Geometry: final body of the model. Coordinates: model frame, mm. A direction names the side the tool comes from. Give positions to 0.01 mm unless a question says otherwise; leave off trailing zeros. Loops run counter-clockwise (first coordinate to the right, second up) from the corner with the lowest first, then second, coordinate; pieces in that order, holes last. Notation, with made-up numbers: (-11, 53) - (2, 53) arc R12 ccw to (2, 69) - close; hole circle Ø1 at (75.5, 48.5). An arc over 180 degrees is marked (long way). Use CSV: the item, a comma, the result in double quotes. Start each with the question number.
```python
from build123d import *

# Parameters (mm, degrees)
BOSS_EXTRU_1_DEPTH      = 6
BOSS_EXTRU_2_DEPTH      = 12
ESQUISSE14_W            = 21
ESQUISSE14_H            = 6
ENL_V_MAT_EXTRU_2_DEPTH = 21
D_GAGEMENT_M81_D        = 9
TROU_TARAUD_M82_D       = 6.8
ESQUISSE19_W            = 31.228123836
ESQUISSE19_H            = 16.033363116
ENL_V_MAT_EXTRU_3_DEPTH = 22
ESQUISSE20_W            = 8
ESQUISSE20_H            = 6
BOSS_EXTRU_3_DEPTH      = 25
BOSS_EXTRU_4_DEPTH      = 6
TROU_TARAUD_M83_D       = 6.8
ESQUISSE25_W            = 25
ESQUISSE25_H            = 6
ENL_V_MAT_EXTRU_4_DEPTH = 3
ENL_V_START             = -13
ENL_V_MAT_EXTRU_5_DEPTH = 14


with BuildPart() as part:
    # Esquisse1 → Boss.-Extru.1 (new body)
    with BuildSketch(Plane(origin=(0, 0, 0), x_dir=(1, 0, 0), z_dir=(0, 1, 0))):
        with BuildLine():
            Line((0, 0), (0, 30))
            ThreePointArc((0, 30), (10, 40), (20, 30))
            Line((20, 30), (20, 0))
            ThreePointArc((20, 0), (10, -10), (0, 0))
        make_face()
    extrude(amount=BOSS_EXTRU_1_DEPTH)

    # Esquisse12 → Boss.-Extru.2 (add)
    with BuildSketch(Plane.XZ):
        with BuildLine():
            Line((0, -30), (20, -30))
            Line((20, -30), (20, 0))
            ThreePointArc((20, 0), (10, 10), (0, 0))
            Line((0, 0), (0, -30))
        make_face()
    extrude(amount=BOSS_EXTRU_2_DEPTH)

    # Esquisse14 → Enlèv. mat.-Extru.2 (cut, through all)
    with BuildSketch(Plane(origin=(20, 0, 0), x_dir=(0, 0, -1), z_dir=(1, 0, 0))):
        with Locations((0.5, 3)):
            Rectangle(ESQUISSE14_W, ESQUISSE14_H)
        Polygon((30, 0), (19, 0), (19, -6), (-10, -6), (-10, -12), (30, -12), align=None)
    extrude(amount=-ENL_V_MAT_EXTRU_2_DEPTH, mode=Mode.SUBTRACT)

    # Dégagement M81 (through all)
    with Locations(Plane(origin=(0, 6, 0), x_dir=(1, 0, 0), z_dir=(0, 1, 0))):
        with Locations((10, 30)):
            Hole(D_GAGEMENT_M81_D / 2)

    # Trou taraudé M82 (through all)
    with Locations(Plane(origin=(0, 0, 0), x_dir=(1, 0, 0), z_dir=(0, 1, 0))):
        with Locations((10, 0)):
            Hole(TROU_TARAUD_M82_D / 2)

    # Esquisse19 → Enlèv. mat.-Extru.3 (cut, through all)
    with BuildSketch(Plane.XY.offset(-11)):
        with Locations((8.695037224, -0.70266631)):
            Rectangle(ESQUISSE19_W, ESQUISSE19_H)
    extrude(amount=ENL_V_MAT_EXTRU_3_DEPTH, mode=Mode.SUBTRACT)

    # Esquisse20 → Boss.-Extru.3 (add)
    with BuildSketch(Plane.ZY):
        with Locations((-15, -3)):
            Rectangle(ESQUISSE20_W, ESQUISSE20_H)
    extrude(amount=BOSS_EXTRU_3_DEPTH)

    # Esquisse21 → Boss.-Extru.4 (add)
    with BuildSketch(Plane.XZ.offset(6)):
        with BuildLine():
            Line((-25, -19), (-25, -30))
            ThreePointArc((-25, -30), (-15, -40), (-5, -30))
            Line((-5, -30), (-5, -19))
            Line((-5, -19), (-25, -19))
        make_face()
    extrude(amount=-BOSS_EXTRU_4_DEPTH)

    # Trou taraudé M83 (through all)
    with Locations(Plane(origin=(0, 0, 0), x_dir=(1, 0, 0), z_dir=(0, 1, 0))):
        with Locations((-15, 30)):
            Hole(TROU_TARAUD_M83_D / 2)

    # Esquisse25 → Enlèv. mat.-Extru.4 (cut)
    with BuildSketch(Plane(origin=(0, 0, -19), x_dir=(-1, 0, 0), z_dir=(0, 0, -1))):
        with Locations((-7.5, -3)):
            Rectangle(ESQUISSE25_W, ESQUISSE25_H)
    extrude(amount=-ENL_V_MAT_EXTRU_4_DEPTH, mode=Mode.SUBTRACT)

    # Esquisse27 → Enlèv. mat.-Extru.5 (cut)
    with BuildSketch(Plane.XZ.offset(6).offset(ENL_V_START)):
        Polygon((-25, -11), (-10, -11), (-25, -23.586494468), align=None)
    enl_v_mat_extru_5 = extrude(amount=ENL_V_MAT_EXTRU_5_DEPTH, mode=Mode.SUBTRACT)

    # Symétrie1: Enlèv. mat.-Extru.5 across plane
    add(enl_v_mat_extru_5.mirror(Plane(origin=(-2.5, 0, 0), x_dir=(0, 0, 1), z_dir=(1, 0, 0))), mode=Mode.SUBTRACT)


solid = part.part
```
Item 1: Pin query (flat end, axial travel): pin 1 Ø5 at (y, z) = (3.5, -20.5) entering from -X; pin 2 Ø11.5 at (x, z) = (10, -30) entering from -Y; pin 3 Ø6.5 at (x, y) = (-0.5, -2) entering from -Z; pin 4 Ø4 at (x, z) = (-15, -30) entering from +Y. Return the tip coordinate at first contact, or that it passes through.
Item 2: Section C-C (y = 1.25). Output: boundary loops of the cut face in (x, z), plus the area to 3 significant figures.
Item 3: Section B-B (y = -4.75). Output: boundary loops of the cut face in (x, z), plus the area to 3 significant figures.
Item 4: Section A-A (x = -12.5). Output: boundary loops of the cut face in (y, z), plus the area to 3 significant figures.
Item 5: Mould query, pull axis Z, two halves, no side actions, for faces 1 (the flat face through (7.9, 0, -25.5)), 2 (the cylindrical face through (-14.26, -3.04, -26.68)), 3 (the flat face through (10.73, 1.42, -15.81)), 4 (the cylindrical face through (10, 3, -40)). Classes: pulls with the +Z half, pulls with the -Z half, needs draft (parallel to the pull), parting line crosses it, or undercut.
Item 6: Reachability of faces 5 (the flat face through (3, -3, -16)), 6 (the flat face through (-13, 0, -25)), 7 (the flat face through (-5, -3, -23)) from +Z, -Z, +X, -X, +Y, -Y: full face, straight path, thin tool, end or side. Return the list, or none.
Item 7: Ray query, probe 1 along X at (y, z) = (2.1, -30); probe 2 along Y at (x, z) = (15, -32.25); probe 3 along Y at (x, z) = (-18, -26.25). Return the intervals inside material, ascending.
Item 8: Section D-D (x = 10). Output: boundary loops of the cut face in (y, z).
Outcome:
1,pin 1,"stops at x = 0"
1,pin 2,"stops at y = 0"
1,pin 3,"stops at z = -36.08"
1,pin 4,"passes through"
2,outline,"(0, -30) arc R10 ccw to (20, -30) - (20, -23.59) - (5, -11) - (0, -11) - close; hole circle Ø9 at (10, -30)"
2,area,"379 mm2"
3,outline,"(-25, -30) arc R10 ccw to (-5, -30) - (-5, -16) - (10.96, -16) - (5, -11) - (-10, -11) - (-25, -23.59) - close; hole circle Ø6.8 at (-15, -30)"
3,area,"471 mm2"
4,outline,"(-6, -39.68) - (0, -39.68) - (0, -32.3) - (-6, -32.3) - close; (-6, -27.7) - (0, -27.7) - (0, -13.1) - (-6, -13.1) - close"
4,area,"132 mm2"
5,face 1,"needs draft"
5,face 2,"undercut"
5,face 3,"pulls with the +Z half"
5,face 4,"pulls with the -Z half"
6,face 5,"-Z, +X, -Y"
6,face 6,"+Z, -Z, -X, +Y"
6,face 7,"-Z, +X, +Y, -Y"
7,probe 1,"x = 0 to 5.5, 14.5 to 20"
7,probe 2,"y = 0 to 6"
7,probe 3,"y = -6 to 0"
8,outline,"(-6, -16) - (0, -16) - (0, -25.5) - (6, -25.5) - (6, -15.2) - (-6, -15.2) - close; (0, -40) - (6, -40) - (6, -34.5) - (0, -34.5) - close"
